Geometry check sheet. Reference: drawing and pictorial views, mm from the part's lowest x, y, z. Round coordinates to 2 decimals unless told otherwise and drop trailing zeros. Order: outer loops, then holes, each group sorted by start corner. A loop starts at its lowest first (then second) coordinate and runs counter-clockwise, first axis right, second up.
(1) Sectioned sample at D-D (z = 1.75). Record the boundary of the cut face in (x, y).
(2) Release check for a two-part mould opening along X. For the marked faces 1 and 2 record: +X half, -X half, draft (parallel to the pull), parting line (faces both ways), or undercut.
(3) Go/stop test with flat-tipped pins: pin 1 (0.5 mm diameter, centred on x = 27, z = 8.5, fed in from -Y); pin 2 (3 mm diameter, centred on y = 6.5, z = 2, fed in from -X); pin 3 (1.8 mm diameter, centred on x = 2.5, z = 8.5, fed in from +Y). Record where each tip stops, or that it passes through.
(4) Material ranges on line 1 along Y through (x, z) = (28, 8.4); line 2 along X through (y, z) = (1.75, 4); line 3 along Z through (x, y) = (3.5, 5), recorded low to high.
(5) Sectioned sample at B-B (y = 5). Record the boundary of the cut face in (x, z), plus the area to 3 significant figures.
(6) Sectioned sample at A-A (x = 28). Record the boundary of the cut face in (y, z), plus the area to 3 significant figures.
(7) Sectioned sample at C-C (z = 8.75). Record the boundary of the cut face in (x, y).
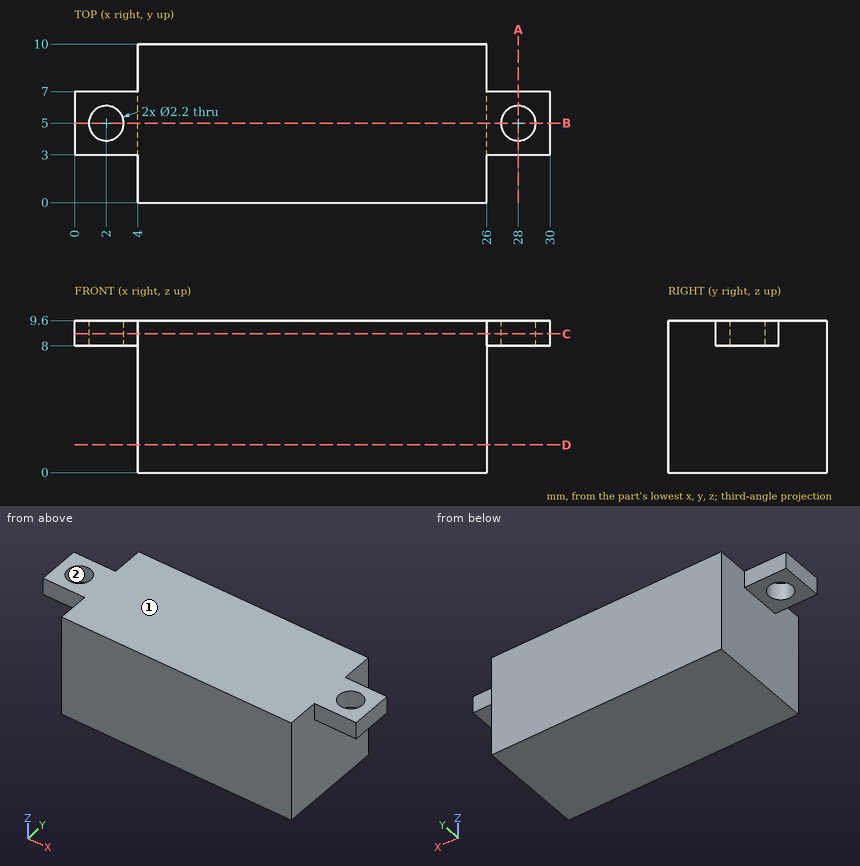
Answer below:
1. outline: (4, 0) - (26, 0) - (26, 10) - (4, 10) - close
2. face 1: draft
2. face 2: undercut
3. pin 1: stops at y = 3
3. pin 2: stops at x = 4
3. pin 3: stops at y = 7
4. line 1: y = 3 to 3.9, 6.1 to 7
4. line 2: x = 4 to 26
4. line 3: z = 8 to 9.6
5. outline: (0, 8) - (0.9, 8) - (0.9, 9.6) - (0, 9.6) - close; (3.1, 8) - (4, 8) - (4, 0) - (26, 0) - (26, 8) - (26.9, 8) - (26.9, 9.6) - (3.1, 9.6) - close; (29.1, 8) - (30, 8) - (30, 9.6) - (29.1, 9.6) - close
5. area: 217 mm2
6. outline: (3, 8) - (3.9, 8) - (3.9, 9.6) - (3, 9.6) - close; (6.1, 8) - (7, 8) - (7, 9.6) - (6.1, 9.6) - close
6. area: 2.88 mm2
7. outline: (0, 3) - (4, 3) - (4, 0) - (26, 0) - (26, 3) - (30, 3) - (30, 7) - (26, 7) - (26, 10) - (4, 10) - (4, 7) - (0, 7) - close; hole circle Ø2.2 at (2, 5); hole circle Ø2.2 at (28, 5)
